The model under review builds one solid part; all positions refer to its coordinate system, in mm. A direction names the side the tool comes from. Round coordinates to 2 decimals unless told otherwise and drop trailing zeros. Write each loop counter-clockwise with the first axis right and the second up, starting at its lowest first coordinate (ties: lowest second). Pieces come first, ordered by that corner, then holes. Notation, with made-up numbers: (69.25, -22.75) -> (111.25, -22.75) arc R19 ccw to (111.25, 10.25) -> close; hole circle Ø3 at (55.5, 18). An arc over 180 degrees is marked (long way). Use CSV: the item, a comma, the result in double quotes. Start each with the question number.
1) Wall thickness on probe 1 along X at (y, z) = (35.55, 0); probe 2 along Y at (x, z) = (-12, 0); probe 3 along Y at (x, z) = (-4, -7): over which ranges is each line inside the solid? List them lowest first. Write a range as [from, to].
2) For pin 1 Ø4 at (y, z) = (37, 0) entering from -X; pin 2 Ø3 at (x, z) = (0.5, 1.5) entering from +Y; pin 3 Ø2.5 at (y, z) = (36.5, 0) entering from +X, all flat-tipped, find the tip position at first contact; note any pin that passes through.
3) Mouldability with a two-part tool opening along Y and no side actions: class faces 3 (the face through (-7.086, 0.751, 17.089)), 4 (the face through (10.967, 41.525, 0.163)), 5 (the face through (0, 37.4, 0)) as released by +Y, released by -Y, zero draft, split by the parting line, or undercut.
4) Take a section at A-A, the plane z = 0. State how many separate pieces and enclosed holes the cut face has, then the cut area to 3 significant figures.
5) Take a section at C-C, the plane y = 32. Give the boundary of the cut face in (x, z).
6) Take a section at B-B, the plane x = 0. Give the boundary of the cut face in (y, z).
7) Take a section at D-D, the plane y = -2. Give the boundary of the cut face in (x, z), then the cut area to 3 significant figures.
8) Machinability: for faces 1 (the face through (11.361, 38, 0)), 2 (the face through (-12.233, 41.525, 0.163)), which of the approach directions +Z, -Z, +X, -X, +Y, -Y give a long, thin tool a straight path to every point of the face, cutting with its end or side? Answer none if there is none.
from build123d import *

# Parameters (mm, degrees)
CROQUIS1_R                = 18.5
SALIENTE_EXTRUIR1_DEPTH   = 18.4
CROQUIS2_R                = 17.9
SALIENTE_EXTRUIR2_DEPTH   = 18
CROQUIS3_R                = 17.3
CORTAR_EXTRUIR1_DEPTH     = 1.5
CROQUIS4_R                = 5
SALIENTE_EXTRUIR3_DEPTH   = 2.5
CROQUIS5_W                = 0.8
CROQUIS5_H                = 5
SALIENTE_EXTRUIR4_DEPTH   = 7
CHAFL_N1_SIZE             = 1
CHAFL_N2_SIZE             = 1
CROQUIS6_R                = 1.25
CORTAR_EXTRUIR2_DEPTH     = 7
MATRIZL1_COUNT            = 2
MATRIZL1_PITCH            = 23.2
CHAFL_N1_OF_MATRIZL1_SIZE = 1
CHAFL_N2_OF_MATRIZL1_SIZE = 1
REDONDEO1_R               = 1


with BuildPart() as part:
    # Croquis1 → Saliente-Extruir1 (new, symmetric)
    with BuildSketch(Plane(origin=(0, 0, 0), x_dir=(1, 0, 0), z_dir=(0, 1, 0))):
        with Locations(Location((0, 0, 0), (0, 0, 270))):
            Circle(CROQUIS1_R)
    extrude(amount=SALIENTE_EXTRUIR1_DEPTH, both=True)

    # Croquis2 → Saliente-Extruir2 (add)
    with BuildSketch(Plane(origin=(0, 18.4, 0), x_dir=(1, 0, 0), z_dir=(0, 1, 0))):
        with Locations(Location((0, 0, 0), (0, 0, 270))):
            Circle(CROQUIS2_R)
    extrude(amount=SALIENTE_EXTRUIR2_DEPTH)

    # Croquis3 → Cortar-Extruir1 (cut)
    with BuildSketch(Plane(origin=(0, 36.4, 0), x_dir=(1, 0, 0), z_dir=(0, 1, 0))):
        with Locations(Location((0, 0, 0), (0, 0, 270))):
            Circle(CROQUIS3_R)
    extrude(amount=-CORTAR_EXTRUIR1_DEPTH, mode=Mode.SUBTRACT)

    # Croquis4 → Saliente-Extruir3 (add)
    with BuildSketch(Plane(origin=(0, 34.9, 0), x_dir=(1, 0, 0), z_dir=(0, 1, 0))):
        with Locations(Location((0, 0, 0), (0, 0, 270))):
            Circle(CROQUIS4_R)
    extrude(amount=SALIENTE_EXTRUIR3_DEPTH)

    # Croquis5 → Saliente-Extruir4 (add)
    with BuildSketch(Plane(origin=(0, 34.9, 0), x_dir=(1, 0, 0), z_dir=(0, 1, 0))):
        with Locations((-12.23891887, 0)):
            Rectangle(CROQUIS5_W, CROQUIS5_H)
    saliente_extruir4 = extrude(amount=SALIENTE_EXTRUIR4_DEPTH)

    # Chaflán1
    chafl_n1_edges = [part.edges().sort_by_distance(p)[0] for p in [
        (-12.23891887, 41.9, 2.5),
    ]]
    chamfer(chafl_n1_edges, length=CHAFL_N1_SIZE)

    # Chaflán2
    chafl_n2_edges = [part.edges().sort_by_distance(p)[0] for p in [
        (-12.23891887, 41.9, -2.5),
    ]]
    chamfer(chafl_n2_edges, length=CHAFL_N2_SIZE)

    # Croquis6 → Cortar-Extruir2 (cut)
    with BuildSketch(Plane(origin=(-11.83891887, 0, 0), x_dir=(0, 0, -1), z_dir=(1, 0, 0))):
        with Locations((0, 40.285474099)):
            Circle(CROQUIS6_R)
    cortar_extruir2 = extrude(amount=-CORTAR_EXTRUIR2_DEPTH, mode=Mode.SUBTRACT)

    # MatrizL1: Saliente-Extruir4, Cortar-Extruir2 ×2
    with Locations(*[(i * MATRIZL1_PITCH, 0, 0) for i in range(1, MATRIZL1_COUNT)]):
        add(saliente_extruir4)
        add(cortar_extruir2, mode=Mode.SUBTRACT)

    # Chaflán1 of MatrizL1
    chafl_n1_of_matrizl1_edges = [part.edges().sort_by_distance(p)[0] for p in [
        (10.96108113, 41.9, 2.5),
    ]]
    chamfer(chafl_n1_of_matrizl1_edges, length=CHAFL_N1_OF_MATRIZL1_SIZE)

    # Chaflán2 of MatrizL1
    chafl_n2_of_matrizl1_edges = [part.edges().sort_by_distance(p)[0] for p in [
        (10.96108113, 41.9, -2.5),
    ]]
    chamfer(chafl_n2_of_matrizl1_edges, length=CHAFL_N2_OF_MATRIZL1_SIZE)

    # Redondeo1
    redondeo1_edges = [part.edges().sort_by_distance(p)[0] for p in [
        (0, -18.4, -18.5),
    ]]
    fillet(redondeo1_edges, radius=REDONDEO1_R)


solid = part.part
Values found:
1,probe 1,"[-17.9, -17.3], [-12.64, -11.84], [-5, 5], [10.56, 11.36], [17.3, 17.9]"
1,probe 2,"[-18.4, 39.04], [41.54, 41.9]"
1,probe 3,"[-18.4, 34.9]"
2,pin 1,"x = -17.9"
2,pin 2,"y = 37.4"
2,pin 3,"x = 17.9"
3,face 3,"zero draft"
3,face 4,"undercut"
3,face 5,"released by +Y"
4,separate pieces,"3"
4,enclosed holes,"0"
4,area,"1,990 mm²"
5,outline,"circle Ø35.8 at (0, 0)"
6,outline,"(-18.4, -17.5) arc R1 ccw to (-17.4, -18.5) -> (18.4, -18.5) -> (18.4, -17.9) -> (36.4, -17.9) -> (36.4, -17.3) -> (34.9, -17.3) -> (34.9, -5) -> (37.4, -5) -> (37.4, 5) -> (34.9, 5) -> (34.9, 17.3) -> (36.4, 17.3) -> (36.4, 17.9) -> (18.4, 17.9) -> (18.4, 18.5) -> (-17.4, 18.5) arc R1 ccw to (-18.4, 17.5) -> close"
7,outline,"circle Ø37 at (0, 0)"
7,area,"1,080 mm²"
8,face 1,"+Y"
8,face 2,"+X, -X"
